from build123d import *

# Parameters (mm, degrees)
SKETCH_1_W                 = 70
SKETCH_1_H                 = 50
EXTRUDE_1_DEPTH            = 40
EXTRUDE_2_DEPTH            = 10
EXTRUDE_2_DEPTH_BACK       = 60
CUT_EXTRUDE_1_REACH        = 108.771
SKETCH_7_W                 = 10
SKETCH_7_H                 = 40
CUT_EXTRUDE_2_DEPTH        = 10
HOLE_WIZARD_M3_2_OUTLINE_R = 1.7
HOLE_WIZARD_M3_2_DEPTH     = 5


# Read off the part's stored shape, not the designer's step: M3 すきま穴1, M3 すきま穴2
with BuildPart() as part:
    # ｽｹｯﾁ1 → ﾎﾞｽ - 押し出し1 (new body)
    with BuildSketch(Plane.XY):
        with Locations((35, 25)):
            Rectangle(SKETCH_1_W, SKETCH_1_H)
    extrude(amount=EXTRUDE_1_DEPTH)

    # ｽｹｯﾁ2 → ﾎﾞｽ - 押し出し2 (add, two sides: drawn at the far end of the back side and taken through both)
    with BuildSketch(Plane(origin=(0, 50, 0), x_dir=(1, 0, 0), z_dir=(0, 1, 0)).offset(-EXTRUDE_2_DEPTH_BACK)):
        Polygon((16, 0), (16, -5), (26, -5), (26, -9), (44, -9), (44, -5), (54, -5), (54, 0), align=None)
    extrude(amount=EXTRUDE_2_DEPTH + EXTRUDE_2_DEPTH_BACK)

    # M3 すきま穴1 outline → M3 すきま穴1 (revolve, cut)
    with BuildSketch(Plane(origin=(49, -5, 0), x_dir=(1, 0, 0), z_dir=(0, -1, 0))):
        Polygon((0, 0), (1.7, 0), (1.7, 4.97124079), (1.725, 5), (0, 5), align=None)
    revolve(axis=Axis((49, -5, 0), (0, 0, 1)), mode=Mode.SUBTRACT)

    # Hole Wizard M3 _1 2 outline → Hole Wizard M3 _1 2 (revolve, cut)
    with BuildSketch(Plane(origin=(21, -5, 0), x_dir=(1, 0, 0), z_dir=(0, -1, 0))):
        Polygon((0, 0), (1.7, 0), (1.7, 4.97124079), (1.725, 5), (0, 5), align=None)
    revolve(axis=Axis((21, -5, 0), (0, 0, 1)), mode=Mode.SUBTRACT)

    # Hole Wizard M3 _1 3 outline → Hole Wizard M3 _1 3 (revolve, cut)
    with BuildSketch(Plane(origin=(49, 55, 0), x_dir=(1, 0, 0), z_dir=(0, -1, 0))):
        Polygon((0, 0), (1.7, 0), (1.7, 4.97124079), (1.725, 5), (0, 5), align=None)
    revolve(axis=Axis((49, 55, 0), (0, 0, 1)), mode=Mode.SUBTRACT)

    # Hole Wizard M3 _1 4 outline → Hole Wizard M3 _1 4 (revolve, cut)
    with BuildSketch(Plane(origin=(21, 55, 0), x_dir=(1, 0, 0), z_dir=(0, -1, 0))):
        Polygon((0, 0), (1.7, 0), (1.7, 4.97124079), (1.725, 5), (0, 5), align=None)
    revolve(axis=Axis((21, 55, 0), (0, 0, 1)), mode=Mode.SUBTRACT)

    # ｽｹｯﾁ6 → ｶｯﾄ - 押し出し1 (cut, up to next)
    with BuildSketch(Plane(origin=(0, 60, 0), x_dir=(1, 0, 0), z_dir=(0, 1, 0)), mode=Mode.PRIVATE) as cut_extrude_1_sk1:
        with BuildLine():
            Line((28.85, 0), (41.15, 0))
            ThreePointArc((41.15, 0), (35, -6.15), (28.85, 0))
        make_face()
    cut_extrude_1_tool1 = extrude(cut_extrude_1_sk1.sketch, amount=-CUT_EXTRUDE_1_REACH, mode=Mode.PRIVATE) & part.part
    add(cut_extrude_1_tool1.solids().sort_by_distance((35, 60, 2.610141))[0], mode=Mode.SUBTRACT)

    # ｽｹｯﾁ7 → ｶｯﾄ - 押し出し2 (cut)
    with BuildSketch(Plane(origin=(70, 0, 0), x_dir=(0, 0, -1), z_dir=(1, 0, 0))):
        with Locations((-35, 25)):
            Rectangle(SKETCH_7_W, SKETCH_7_H)
    cut_extrude_2 = extrude(amount=-CUT_EXTRUDE_2_DEPTH, mode=Mode.SUBTRACT)

    # ﾐﾗｰ1: ｶｯﾄ - 押し出し2 across plane
    add(cut_extrude_2.mirror(Plane.ZY.offset(-35)), mode=Mode.SUBTRACT)

    # M3 すきま穴2 outline → M3 すきま穴2 (cut)
    with BuildSketch(Plane(origin=(0, 0, 0), x_dir=(1, 0, 0), z_dir=(0, 1, 0))):
        with Locations((65, -35)):
            Circle(HOLE_WIZARD_M3_2_OUTLINE_R)
        with Locations((5, -35)):
            Circle(HOLE_WIZARD_M3_2_OUTLINE_R)
    extrude(amount=HOLE_WIZARD_M3_2_DEPTH, mode=Mode.SUBTRACT)

    # Hole Wizard M3 _2 2 outline → Hole Wizard M3 _2 2 (revolve, cut)
    with BuildSketch(Plane(origin=(65, 0, 35), x_dir=(1, 0, 0), z_dir=(0, 0, 1))):
        Polygon((1.725, 50), (0, 50), (0, 45), (1.7, 45), (1.7, 49.97124079), align=None)
    revolve(axis=Axis((65, 0, 35), (0, 1, 0)), mode=Mode.SUBTRACT)

    # Hole Wizard M3 _2 3 outline → Hole Wizard M3 _2 3 (revolve, cut)
    with BuildSketch(Plane(origin=(5, 0, 35), x_dir=(1, 0, 0), z_dir=(0, 0, 1))):
        Polygon((0, 45), (1.7, 45), (1.7, 49.97124079), (1.725, 50), (0, 50), align=None)
    revolve(axis=Axis((5, 0, 35), (0, 1, 0)), mode=Mode.SUBTRACT)


solid = part.part
Build history of the part. All positions in model axes, mm. A direction names the side the tool comes from. Round coordinates to 2 decimals unless told otherwise and drop trailing zeros. Write each loop counter-clockwise with the first axis right and the second up, starting at its lowest first coordinate (ties: lowest second). Pieces come first, ordered by that corner, then holes. Notation, with made-up numbers: (54, 81) -> (104, 81) arc R27 cw to (104, 98) -> close; hole circle Ø8 at (17.25, 65.25). An arc over 180 degrees is marked (long way). Write item = value, one per line.
(1) Band-saw the part on A-A (y = 55). Give the cut face in (x, z) (3 decimals).
Answer:
outline = (16, 0) -> (19.3, 0) -> (19.3, 4.971) -> (19.275, 5) -> (16, 5) -> close; (22.7, 0) -> (28.85, 0) arc R6.15 cw to (41.15, 0) -> (47.3, 0) -> (47.3, 4.971) -> (47.275, 5) -> (44, 5) -> (44, 9) -> (26, 9) -> (26, 5) -> (22.725, 5) -> (22.7, 4.971) -> close; (50.7, 0) -> (54, 0) -> (54, 5) -> (50.725, 5) -> (50.7, 4.971) -> close
(2) Band-saw the part on B-B (z = 35). State how many separate pieces and enclosed holes the cut face has, then the cut area to 3 significant figures.
Answer:
separate_pieces = 5
enclosed_holes = 0
area = 2,630 mm2
(3) Band-saw the part on D-D (x = 35). Give the cut face in (y, z).
Answer:
outline = (-10, 6.15) -> (60, 6.15) -> (60, 9) -> (50, 9) -> (50, 40) -> (0, 40) -> (0, 9) -> (-10, 9) -> close
(4) Probe L1, parallel to Y at x = 21, z = 2; L2, parallel to X at y = 47, z = 35; L3, parallel to Z at x = 65, y = 3. List the from-to ranges inside material, lowest first.
Answer:
L1 = -10 to -6.7, -3.3 to 53.3, 56.7 to 60
L2 = 0 to 3.3, 6.7 to 63.3, 66.7 to 70
L3 = 0 to 33.3, 36.7 to 40
(5) Band-saw the part on C-C (x = 49). Give the cut face in (y, z) (3 decimals), then the cut area to 3 significant figures.
Answer:
outline = (-10, 0) -> (-6.7, 0) -> (-6.7, 4.971) -> (-6.725, 5) -> (-10, 5) -> close; (-3.3, 0) -> (53.3, 0) -> (53.3, 4.971) -> (53.275, 5) -> (50, 5) -> (50, 40) -> (0, 40) -> (0, 5) -> (-3.275, 5) -> (-3.3, 4.971) -> close; (56.7, 0) -> (60, 0) -> (60, 5) -> (56.725, 5) -> (56.7, 4.971) -> close
area = 2,070 mm2
(6) Flat gauge pins, fed straight in: pin 1 (8 mm diameter, centred on x = 23, y = 55, fed in from +Z); pin 2 (20 mm diameter, centred on x = 22.5, z = 18.5, fed in from +Y); pin 3 (3 mm diameter, centred on y = 12, z = 35.5, fed in from +X); pin 4 (8 mm diameter, centred on y = 36.5, z = 17.5, fed in from -X). Where does each tip first touch, or does it go through?
Answer:
pin_1 = 9
pin_2 = 50
pin_3 = 60
pin_4 = 0
(7) Two-plate mould, pull along Y, no slides. Class faces 6 (the face through (34.7, -10, 6.4)), 7 (the face through (65, 25, 30)), 8 (the face through (4.63, 2.46, 36.66)): pulls with the +Y half, pulls with the -Y half, needs draft (parallel to the pull), parting line crosses it, or undercut.
Answer:
face_6 = pulls with the -Y half
face_7 = undercut
face_8 = needs draft
(8) Tool access for faces 1 (the face through (54, -5, 3)), 2 (the face through (35, 55, 9)), 3 (the face through (54, 55, 3)), 4 (the face through (5, 5, 33)), 5 (the face through (44, 55, 7)): list every direction of +Z, -Z, +X, -X, +Y, -Y with a clear straight run to the whole face (end or side of a thin tool).
Answer:
face_1 = +Z, -Z, +X, -Y
face_2 = +Z, +X, -X, +Y
face_3 = +Z, -Z, +X, +Y
face_4 = +Z, -X
face_5 = +Z, +X, +Y
